Verification items for the finished model (mm, model axes). Give positions to 0.01 mm unless a question says otherwise; leave off trailing zeros. Write each loop counter-clockwise with the first axis right and the second up, starting at its lowest first coordinate (ties: lowest second). Pieces come first, ordered by that corner, then holes. Notation, with made-up numbers: (-14, 3.5) - (22, 3.5) arc R30 cw to (22, 41.5) - close; hole circle Ø1 at (-3, 25). An arc over 180 degrees is marked (long way). Answer as a JSON object with one key per item and string values. Group by question number.
Item 1: Draft check along Y on faces 1 (the face through (0, 30, 10)), 2 (the face through (80.968, 79.127, 9.86)), 3 (the face through (34.614, 36.128, 9.86)). Enter one of: +Y half, -Y half, draft (parallel to the pull), parting line (faces both ways), or undercut.
Item 2: Sectioned sample at B-B, the plane y = 30. Record the boundary of the cut face in (x, z).
Item 3: Go/stop test with flat-tipped pins: pin 1 (10 mm diameter, centred on x = 82, y = 11, fed in from -Z); pin 2 (1 mm diameter, centred on x = 49.5, z = 5.5, fed in from +Y); pin 3 (2 mm diameter, centred on y = 48.5, z = 12.5, fed in from +X); pin 4 (3 mm diameter, centred on y = 19, z = 14.5, fed in from +X). Record where each tip stops, or that it passes through.
Item 4: Sectioned sample at A-A, the plane x = 29.5. Record the boundary of the cut face in (y, z), and give its area (3 significant figures).
Item 5: Sectioned sample at D-D, the plane y = 10.5. Record the boundary of the cut face in (x, z), and give its area (3 significant figures).
Item 6: Sectioned sample at C-C, the plane z = 17.75. Record the boundary of the cut face in (x, y).
Item 7: Scan lines: line 1 along X through (y, z) = (36, 9.75); line 2 along X through (y, z) = (21.5, 1.5); line 3 along Y through (x, z) = (82, 12.75). Record each from-to range of solid material in increasing order. Write a range as [from, to].
```python
from build123d import *

# Parameters (mm, degrees)
F0_R     = 10
F1_DEPTH = 20


with BuildPart() as f1:
    # F0 (on Top) → F1 (new body)
    with BuildSketch(Plane.XY):
        with BuildLine():
            Line((0, 60), (0, 0))
            Line((0, 0), (100, 0))
            ThreePointArc((100, 0), (79.878387, 79.797312), (0, 60))
        make_face()
        with Locations((80, 30)):
            Circle(F0_R, mode=Mode.SUBTRACT)
        with Locations((30, 45)):
            Circle(F0_R, mode=Mode.SUBTRACT)
    extrude(amount=F1_DEPTH)


solid = f1.part
```
Geometry check:
{
 "1": {"face 1": "draft", "face 2": "parting line", "face 3": "undercut"},
 "2": {"outline": "(0, 0) - (70, 0) - (70, 20) - (0, 20) - close; (90, 0) - (108.19, 0) - (108.19, 20) - (90, 20) - close"},
 "3": {"pin 1": "z = 0", "pin 2": "y = 88.11", "pin 3": "x = 105.44", "pin 4": "x = 107.44"},
 "4": {"outline": "(0, 0) - (35.01, 0) - (35.01, 20) - (0, 20) - close; (54.99, 0) - (84.43, 0) - (84.43, 20) - (54.99, 20) - close", "area": "1,290 mm^2"},
 "5": {"outline": "(0, 0) - (104.9, 0) - (104.9, 20) - (0, 20) - close", "area": "2,100 mm^2"},
 "6": {"outline": "(0, 0) - (100, 0) arc R58.31 ccw to (0, 60) - close; hole circle Ø20 at (30, 45); hole circle Ø20 at (80, 30)"},
 "7": {"line 1": "[0, 25.64], [34.36, 72], [88, 107.86]", "line 2": "[0, 74.73], [85.27, 107.59]", "line 3": "[0, 20.2], [39.8, 78.46]"}
}
